Could you check a few things on this drawing? It's one solid part, dimensions in mm from its lowest x, y, z. A direction names the side the tool comes from. Give positions to 0.01 mm unless a question says otherwise; leave off trailing zeros. Loops run counter-clockwise (first coordinate to the right, second up) from the corner with the lowest first, then second, coordinate; pieces in that order, holes last.
1. Imagine slicing it at D-D (y = 9.25). List the corners of the cut face in (x, z) for me.
2. Imagine slicing it at C-C (x = 11.25). List the corners of the cut face in (y, z) for me, plus the area to 3 significant figures.
3. For the marked faces 1, 2 and 3, which set-ups out of +Z, -Z, +X, -X, +Y, -Y let a thin tool reach every point of the face, with its end or its side?
4. I need wall thicknesses on line 1 along X through (y, z) = (8.5, 3); line 2 along Y through (x, z) = (10.5, 4); line 3 along Z through (x, y) = (7.25, 1). Which ranges of each line are inside material? Lowest first, please.
5. For P1, Ø3, axis at x = 10.5, y = 8.5, coming from the +Z side; P2, Ø3, axis at x = 5, y = 3.5, coming from the -Z side; P3, Ø5, axis at y = 1.5, z = 1.5, coming from the +X side; P4, Ø1.5, axis at x = 11.5, y = 8.5, coming from the +Z side, each with a flat end and sliding along its axis, tell me the tip position at first contact or that it passes through.
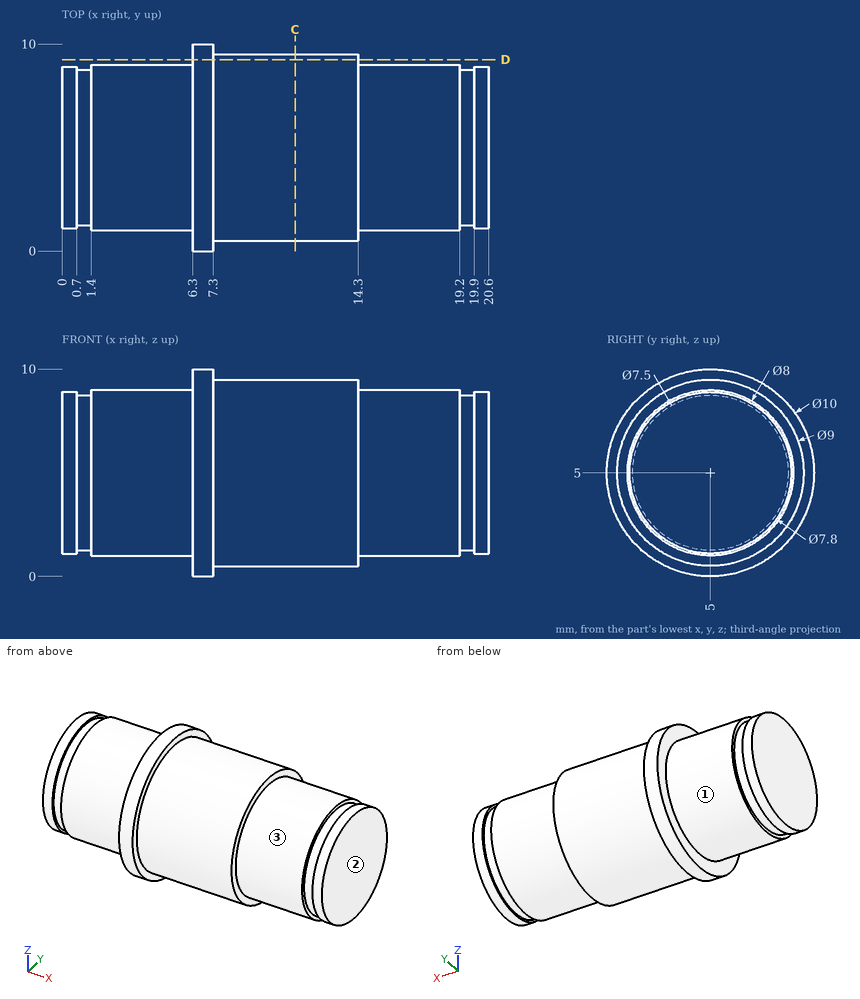
Derived:
1. outline: (6.3, 2.37) - (7.3, 2.37) - (7.3, 3.52) - (14.3, 3.52) - (14.3, 6.48) - (7.3, 6.48) - (7.3, 7.63) - (6.3, 7.63) - close
2. outline: circle Ø9 at (5, 5)
2. area: 63.6 mm2
3. face 1: -X
3. face 2: +Z, -Z, +X, +Y, -Y
3. face 3: +X
4. line 1: x = 6.3 to 14.3
4. line 2: y = 0.61 to 9.39
4. line 3: z = 2 to 8
5. P1: stops at z = 9.03
5. P2: stops at z = 0.06
5. P3: stops at x = 20.6
5. P4: stops at z = 8.56
